Verification items for the finished model (mm, model axes). Face numbers are marked on the shaded views. A direction names the side the tool comes from. Coordinates: 2 decimals unless noted, no trailing zeros. Write each loop counter-clockwise with the first axis right and the second up, starting at its lowest first coordinate (ties: lowest second). Pieces come first, ordered by that corner, then holes. Notation, with made-up numbers: (12.5, 11) -> (43.5, 11) arc R21 ccw to (43.5, 24) -> close; hole circle Ø5 at (22.5, 83.5). An arc over 180 degrees is marked (long way). Answer in a Markdown table with one row per item.
```python
from build123d import *

# Parameters (mm, degrees)
SKETCH1_W           = 10.2
SKETCH1_H           = 7
BOSS_EXTRUDE1_DEPTH = 15
SKETCH2_W           = 10
SKETCH2_H           = 12
BOSS_EXTRUDE2_DEPTH = 9
FILLET1_R           = 0.508
SKETCH3_W           = 10
SKETCH3_H           = 6.9
BOSS_EXTRUDE3_DEPTH = 0.57
SKETCH4_R           = 1.5
CUT_EXTRUDE1_DEPTH  = 8.952


with BuildPart() as part:
    # Sketch1 → Boss-Extrude1 (new body)
    with BuildSketch(Plane(origin=(0, 0, 0), x_dir=(1, 0, 0), z_dir=(0, 1, 0))):
        with BuildLine():
            Line((-5.1, -3.5), (5.1, -3.5))
            ThreePointArc((5.1, -3.5), (0, -6), (-5.1, -3.5))
        make_face()
        Rectangle(SKETCH1_W, SKETCH1_H)
        with BuildLine():
            ThreePointArc((-5.1, 3.5), (0, 6), (5.1, 3.5))
            Line((5.1, 3.5), (-5.1, 3.5))
        make_face()
    extrude(amount=BOSS_EXTRUDE1_DEPTH)

    # Sketch2 → Boss-Extrude2 (add)
    with BuildSketch(Plane(origin=(0, 15, 0), x_dir=(1, 0, 0), z_dir=(0, 1, 0))):
        Rectangle(SKETCH2_W, SKETCH2_H)
    extrude(amount=BOSS_EXTRUDE2_DEPTH)

    # Fillet1
    fillet1_edges = [part.edges().sort_by_distance(p)[0] for p in [
        (5, 19.5, 6),
        (5, 19.5, -6),
        (-5, 19.5, -6),
        (-5, 19.5, 6),
    ]]
    fillet(fillet1_edges, radius=FILLET1_R)

    # Sketch3 → Boss-Extrude3 (add)
    with BuildSketch(Plane.XZ):
        Rectangle(SKETCH3_W, SKETCH3_H)
        with BuildLine():
            Line((5, -3.45), (-5, -3.45))
            ThreePointArc((-5, -3.45), (0, -5.95), (5, -3.45))
        make_face()
        with BuildLine():
            ThreePointArc((5, 3.45), (0, 5.95), (-5, 3.45))
            Line((-5, 3.45), (5, 3.45))
        make_face()
    extrude(amount=BOSS_EXTRUDE3_DEPTH)

    # Sketch4 → Cut-Extrude1 (cut)
    with BuildSketch(Plane(origin=(0, 24, 0), x_dir=(1, 0, 0), z_dir=(0, 1, 0))):
        with Locations(Location((0, 0, 0), (0, 0, 270))):
            Circle(SKETCH4_R)
    extrude(amount=-CUT_EXTRUDE1_DEPTH, mode=Mode.SUBTRACT)


solid = part.part
```
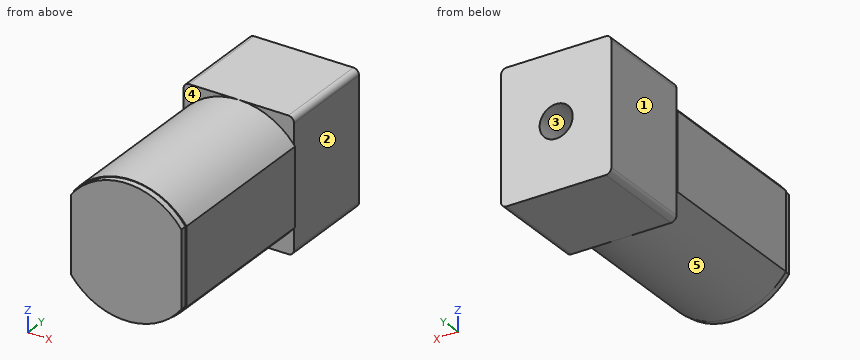
1. Thickness scan on line 1 (X direction, y = 19.5, z = 0); line 2 (Y direction, x = -0.5, z = 0.5); line 3 (Z direction, x = -0.25, y = 3.25). Record the ranges inside material, lowest first. Write a range as from..to.
Geometry says:
| item | result |
|---|---|
| line 1 | -5..-1.5, 1.5..5 |
| line 2 | -0.57..15.05 |
| line 3 | -6..6 |
2. Section check A-A, the plane y = 18.75. Record the boundary of the cut face in (x, z).
Geometry says:
| item | result |
|---|---|
| outline | (-5, -5.49) arc R0.51 ccw to (-4.49, -6) -> (4.49, -6) arc R0.51 ccw to (5, -5.49) -> (5, 5.49) arc R0.51 ccw to (4.49, 6) -> (-4.49, 6) arc R0.51 ccw to (-5, 5.49) -> close; hole circle Ø3 at (0, 0) |
3. Depth check by flat-ended pin: P1, Ø4.5, axis at y = 18.5, z = -0.5, coming from the +X side; P2, Ø6, axis at y = 15, z = 4, coming from the +X side; P3, Ø7, axis at y = 19, z = -2.5, coming from the -X side; P4, Ø1.5, axis at y = 10.5, z = -4.5, coming from the -X side. Enter the tip coordinate at first touch or a pass-through.
Geometry says:
| item | result |
|---|---|
| P1 | x = 5 |
| P2 | x = 5.1 |
| P3 | x = -5 |
| P4 | x = -4.9 |
4. Section check D-D, the plane y = 4.25. Record the boundary of the cut face in (x, z).
Geometry says:
| item | result |
|---|---|
| outline | (-5.1, -3.5) arc R6.45 ccw to (5.1, -3.5) -> (5.1, 3.5) arc R6.45 ccw to (-5.1, 3.5) -> close |
5. Tool access check on the marked faces 1, 2, 3, 4 and 5. Record the directions out of +Z, -Z, +X, -X, +Y, -Y that give a thin tool (end or side, any length) a straight path to the whole face; none if there is none.
Geometry says:
| item | result |
|---|---|
| face 1 | +Z, -Z, -X, +Y |
| face 2 | +Z, -Z, +X, +Y |
| face 3 | +Y |
| face 4 | +Z, -X, -Y |
| face 5 | -Z, -Y |
6. Section check B-B, the plane z = 0. Record the boundary of the cut face in (x, y), plus the area to 3 significant figures.
Geometry says:
| item | result |
|---|---|
| outline | (-5.1, 0) -> (-5, 0) -> (-5, -0.57) -> (5, -0.57) -> (5, 0) -> (5.1, 0) -> (5.1, 15) -> (5, 15) -> (5, 24) -> (1.5, 24) -> (1.5, 15.05) -> (-1.5, 15.05) -> (-1.5, 24) -> (-5, 24) -> (-5, 15) -> (-5.1, 15) -> close |
| area | 222 mm^2 |
7. Section check C-C, the plane x = -0.75. Record the boundary of the cut face in (y, z).
Geometry says:
| item | result |
|---|---|
| outline | (-0.57, -5.9) -> (0, -5.9) -> (0, -5.96) -> (15, -5.96) -> (15, -6) -> (24, -6) -> (24, -1.3) -> (15.05, -1.3) -> (15.05, 1.3) -> (24, 1.3) -> (24, 6) -> (15, 6) -> (15, 5.96) -> (0, 5.96) -> (0, 5.9) -> (-0.57, 5.9) -> close |
